Geometry check sheet. Reference: the model listing, model coordinates, mm. Face numbers are marked on the shaded views. Coordinates: 2 decimals unless noted, no trailing zeros. Order: outer loops, then holes, each group sorted by start corner. A loop starts at its lowest first (then second) coordinate and runs counter-clockwise, first axis right, second up. Notation, with made-up numbers: (41.5, 86) -> (53.5, 86) arc R8 ccw to (53.5, 99) -> close; hole circle Ø2 at (58.25, -24). An arc over 180 degrees is marked (long way). Answer in a Markdown table with one row per item. Add a question column.
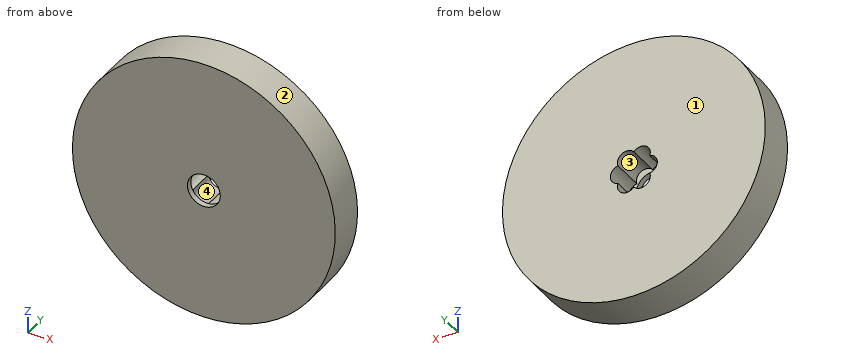
```python
from build123d import *

# Parameters (mm, degrees)
SKETCH1_R           = 100
BOSS_EXTRUDE1_DEPTH = 29
SKETCH2_R           = 12.5
CUT_EXTRUDE1_DEPTH  = 145.364122967
SKETCH3_R           = 7.089633459
CUT_EXTRUDE2_DEPTH  = 24.608661
CIRPATTERN1_START   = 4.391339469
CIRPATTERN1_DEPTH   = 24.608660531


# Read off the part's stored shape, not the designer's step: CirPattern1
with BuildPart() as part:
    # Sketch1 → Boss-Extrude1 (new body)
    with BuildSketch(Plane(origin=(0, 0, 0), x_dir=(1, 0, 0), z_dir=(0, 1, 0))):
        with Locations(Location((0, 0, 0), (0, 0, 90))):
            Circle(SKETCH1_R)
    extrude(amount=BOSS_EXTRUDE1_DEPTH)

    # Sketch2 → Cut-Extrude1 (cut, through all)
    with BuildSketch(Plane(origin=(0, 0, 0), x_dir=(1, 0, 0), z_dir=(0, 1, 0))):
        with Locations(Location((0, 0, 0), (0, 0, 90))):
            Circle(SKETCH2_R)
    extrude(amount=CUT_EXTRUDE1_DEPTH, mode=Mode.SUBTRACT)

    # Sketch3 → Cut-Extrude2 (cut)
    with BuildSketch(Plane(origin=(0, 29, 0), x_dir=(1, 0, 0), z_dir=(0, 1, 0))):
        with Locations((-10.794655518, 0)):
            Circle(SKETCH3_R)
    extrude(amount=-CUT_EXTRUDE2_DEPTH, mode=Mode.SUBTRACT)

    # CirPattern1 outline → CirPattern1 (cut)
    with BuildSketch(Plane(origin=(0, 0, 0), x_dir=(1, 0, 0), z_dir=(0, 1, 0)).offset(CIRPATTERN1_START)):
        with BuildLine():
            ThreePointArc((-10.306567208, -7.072812198), (-11.194950872, -7.078323687), (-12.077048877, -6.97268742))
            ThreePointArc((-12.077048877, -6.97268742), (-8.942144489, -15.488248583), (0, -13.945374841))
            ThreePointArc((0, -13.945374841), (8.942144489, -15.488248583), (12.077048877, -6.97268742))
            ThreePointArc((12.077048877, -6.97268742), (17.884288977, 0), (12.077048877, 6.97268742))
            ThreePointArc((12.077048877, 6.97268742), (8.942144489, 15.488248583), (0, 13.945374841))
            ThreePointArc((0, 13.945374841), (-8.942144489, 15.488248583), (-12.077048877, 6.97268742))
            ThreePointArc((-12.077048877, 6.97268742), (-11.194950872, 7.078323687), (-10.306567208, 7.072812198))
            ThreePointArc((-10.306567208, 7.072812198), (12.5, 0), (-10.306567208, -7.072812198))
        make_face()
    extrude(amount=CIRPATTERN1_DEPTH, mode=Mode.SUBTRACT)


solid = part.part
```
(1) Cross-section at A-A (z = 0). Enter the section's corners in (x, y).
(2) Cross-section at B-B (x = 7.5). Enter the section's corners in (y, z), plus the area to 3 significant figures.
(3) Mould release check, pull along X, two halves, no side actions. Record for the marked faces 1, 2, 3 and 4: +X half, -X half, draft (parallel to the pull), parting line (faces both ways), or undercut.
(4) Scan lines: line 1 along X through (y, z) = (3.4, 0); line 2 along Z through (x, y) = (-8.5, 25.5); line 3 along Z through (x, y) = (8, 1.5). Record each from-to range of solid material in increasing order.
(5) Cross-section at D-D (x = -43). Enter the section's corners in (y, z), plus the area to 3 significant figures.
(6) Cross-section at C-C (y = 12.5). Enter the section's corners in (x, z).
(7) Go/stop test with flat-tipped pins: P1, Ø8.5, axis at x = -13, z = 0.5, coming from the +Y side; P2, Ø5, axis at x = 50, y = 5.5, coming from the +Z side; P3, Ø8, axis at y = 24.5, z = -47, coming from the -X side. Record where each tip stops, or that it passes through.
Checks:
| question | item | result |
|---|---|---|
| 1 | outline | (-100, 0) -> (-12.5, 0) -> (-12.5, 4.39) -> (-17.88, 4.39) -> (-17.88, 29) -> (-100, 29) -> close; (12.5, 0) -> (100, 0) -> (100, 29) -> (17.88, 29) -> (17.88, 4.39) -> (12.5, 4.39) -> close |
| 2 | outline | (0, -99.72) -> (29, -99.72) -> (29, -16.12) -> (4.39, -16.12) -> (4.39, -10) -> (0, -10) -> close; (0, 10) -> (4.39, 10) -> (4.39, 16.12) -> (29, 16.12) -> (29, 99.72) -> (0, 99.72) -> close |
| 2 | area | 4,900 mm² |
| 3 | face 1 | draft |
| 3 | face 2 | parting line |
| 3 | face 3 | undercut |
| 3 | face 4 | undercut |
| 4 | line 1 | -100 to -12.5, 12.5 to 100 |
| 4 | line 2 | -99.64 to -15.72, 15.72 to 99.64 |
| 4 | line 3 | -99.68 to -9.6, 9.6 to 99.68 |
| 5 | outline | (0, -90.28) -> (29, -90.28) -> (29, 90.28) -> (0, 90.28) -> close |
| 5 | area | 5,240 mm² |
| 6 | outline | circle Ø200 at (0, 0); hole (-12.08, -6.97) arc R7.09 ccw to (0, -13.95) arc R7.09 ccw to (12.08, -6.97) arc R7.09 ccw to (12.08, 6.97) arc R7.09 ccw to (0, 13.95) arc R7.09 ccw to (-12.08, 6.97) arc R7.09 ccw to start |
| 7 | P1 | y = 4.39 |
| 7 | P2 | z = 88 |
| 7 | P3 | x = -90.28 |
